from build123d import *

# Parameters (mm, degrees)
F0_W     = 609.6
F0_H     = 609.6
F1_DEPTH = 0.79375
F2_R     = 7.14375
F3_DEPTH = 25.4
F4_R     = 4.7625
F5_DEPTH = 25.4
F6_R     = 6.35
F7_DEPTH = 25.4


# Not quite as in the source:
# - a feature names something its author has since deleted; it is built from what else it names


with BuildPart() as f1:
    # F0 (on Top) → F1 (new body)
    with BuildSketch(Plane.XY):
        with Locations((304.8, 304.8)):
            Rectangle(F0_W, F0_H)
    extrude(amount=F1_DEPTH)

    # F2 (on face) → F3 (cut)
    with BuildSketch(Plane.XY.offset(0.79375)):
        with Locations((187.325, 34.925)):
            Circle(F2_R)
        with Locations((117.475, 50.8)):
            Circle(F2_R)
        with Locations((152.4, 101.6)):
            Circle(F2_R)
        with Locations((152.4, 184.15)):
            Circle(F2_R)
        with Locations((152.4, 288.925)):
            Circle(F2_R)
        with Locations((457.2, 288.925)):
            Circle(F2_R)
        with Locations((457.2, 184.15)):
            Circle(F2_R)
        with Locations((457.2, 101.6)):
            Circle(F2_R)
        with Locations((422.275, 50.8)):
            Circle(F2_R)
        with Locations((492.125, 34.925)):
            Circle(F2_R)
    extrude(amount=-F3_DEPTH, mode=Mode.SUBTRACT)

    # F4 (on face) → F5 (cut)
    with BuildSketch(Plane.XY.offset(0.79375)):
        with Locations((234.95, 558.8)):
            Circle(F4_R)
        with Locations((234.95, 533.4)):
            Circle(F4_R)
        with Locations((374.65, 533.4)):
            Circle(F4_R)
        with Locations((374.65, 558.8)):
            Circle(F4_R)
    extrude(amount=-F5_DEPTH, mode=Mode.SUBTRACT)

    # F6 (on face) → F7 (cut)
    with BuildSketch(Plane(origin=(0, 0, 0), x_dir=(1, 0, 0), z_dir=(0, 0, -1))):
        with Locations((566.7375, -381)):
            Circle(F6_R)
        with Locations((566.7375, -228.6)):
            Circle(F6_R)
    extrude(amount=-F7_DEPTH, mode=Mode.SUBTRACT)


solid = f1.part
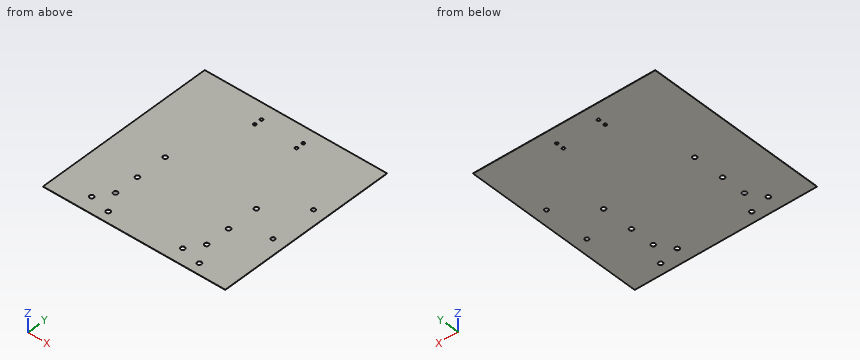
Check sheet for the modelled part. Datum: model origin and axes. Units: mm. Coordinates: 2 decimals unless noted, no trailing zeros. Write each loop counter-clockwise with the first axis right and the second up, starting at its lowest first coordinate (ties: lowest second). Pieces come first, ordered by that corner, then holes.
Item 1: Cross-section at B-B on y = 184.15. Record the boundary of the cut face in (x, z).
Numbers:
outline: (0, 0) - (145.26, 0) - (145.26, 0.79) - (0, 0.79) - close; (159.54, 0) - (450.06, 0) - (450.06, 0.79) - (159.54, 0.79) - close; (464.34, 0) - (609.6, 0) - (609.6, 0.79) - (464.34, 0.79) - close
Item 2: Cross-section at A-A on x = 152.4. Record the boundary of the cut face in (y, z).
Numbers:
outline: (0, 0) - (94.46, 0) - (94.46, 0.79) - (0, 0.79) - close; (108.74, 0) - (177.01, 0) - (177.01, 0.79) - (108.74, 0.79) - close; (191.29, 0) - (281.78, 0) - (281.78, 0.79) - (191.29, 0.79) - close; (296.07, 0) - (609.6, 0) - (609.6, 0.79) - (296.07, 0.79) - close
Item 3: Scan lines: probe 1 along X at (y, z) = (533.4, 0.25); probe 2 along Y at (x, z) = (374.65, 0.65); probe 3 along Y at (x, z) = (152.4, 0.3). Record each from-to range of solid material in increasing order.
Numbers:
probe 1: x = 0 to 230.19, 239.71 to 369.89, 379.41 to 609.6
probe 2: y = 0 to 528.64, 538.16 to 554.04, 563.56 to 609.6
probe 3: y = 0 to 94.46, 108.74 to 177.01, 191.29 to 281.78, 296.07 to 609.6
Item 4: Depth check by flat-ended pin: pin 1 Ø13 at (x, y) = (152.4, 101.6) entering from -Z; pin 2 Ø23 at (x, y) = (457.2, 184.15) entering from -Z. Enter the tip coordinate at first touch or a pass-through.
Numbers:
pin 1: passes through
pin 2: stops at z = 0
